Verification items for the finished model (mm, model axes). Coordinates: 2 decimals unless noted, no trailing zeros. Order: outer loops, then holes, each group sorted by start corner. A loop starts at its lowest first (then second) coordinate and runs counter-clockwise, first axis right, second up. Notation, with made-up numbers: M 43,-31 L 73,-31 A32 cw 73,-1 Z; hole C 68,43.5 d10. An arc over 180 degrees is marked long. Return JSON: item names as keys, results as strings. Group by question number.
Q1. Go/stop test with flat-tipped pins: pin 1 Ø1.8 at (y, z) = (-17, 348) entering from +X; pin 2 Ø1.3 at (y, z) = (-17, 348) entering from -X; pin 3 Ø1.3 at (x, y) = (-2.5, -16.5) entering from -Z. Record where each tip stops, or that it passes through.
Q2. Thickness scan on probe 1 along X at (y, z) = (-6.5, 83); probe 2 along Y at (x, z) = (2, 334). Record the ranges inside material, lowest first.
Q3. Section check B-B, the plane y = 7. Enter the section's corners in (x, z), then the cut area to 3 significant figures.
Q4. Section check A-A, the plane x = -3. Enter the section's corners in (y, z).
Q5. Section check C-C, the plane z = 30. Enter the section's corners in (x, y), then the cut area to 3 significant figures.
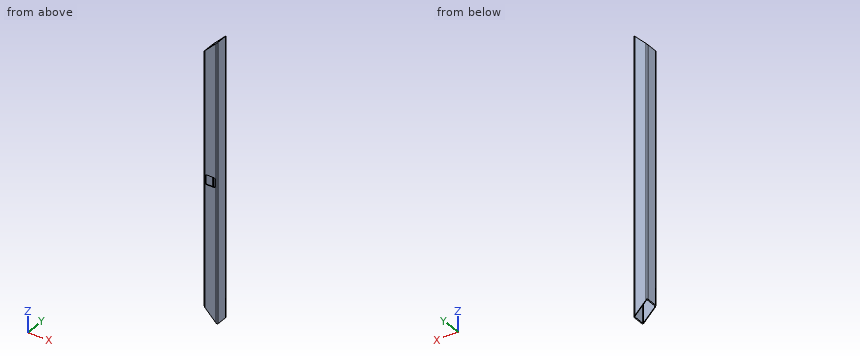
Autodesk Inventor part; units mm, degrees
ref_plane "Start plane" through (0, 0, -17.5) normal (0, 0, 1) x (1, 0, 0)
ref_plane "End plane" through (0, 0, 705.5) normal (0, 0, 1) x (1, 0, 0)
ref_plane "Work Plane4" through (0, 0, 344) normal (0, -1, 0) x (1, 0, 0)
ref_plane "Start plane" through (0, 0, -17.5) normal (0, 0, 1) x (1, 0, 0)
ref_plane "End plane" through (0, 0, 705.5) normal (0, 0, 1) x (1, 0, 0)
sketch "Sketch" plane through (0, 0, 0) normal (0, 0, 1) x (1, 0, 0)
  line L0 (-17.5, -14.3) -> (-17.5, 14.3)
  line L1 (-14.3, 17.5) -> (14.3, 17.5)
  line L2 (17.5, 14.3) -> (17.5, -14.3)
  line L3 (14.3, -17.5) -> (-14.3, -17.5)
  arc A0 (-17.5, -14.3) -> (-14.3, -17.5) centre (-14.3, -14.3) ccw
  arc A1 (-14.3, 17.5) -> (-17.5, 14.3) centre (-14.3, 14.3) ccw
  arc A2 (17.5, 14.3) -> (14.3, 17.5) centre (14.3, 14.3) ccw
  arc A3 (14.3, -17.5) -> (17.5, -14.3) centre (14.3, -14.3) ccw
  arc A4 (-14.3, 15.9) -> (-15.9, 14.3) centre (-14.3, 14.3) ccw
  line L4 (-14.3, 15.9) -> (14.3, 15.9)
  arc A5 (15.9, 14.3) -> (14.3, 15.9) centre (14.3, 14.3) ccw
  line L5 (15.9, 14.3) -> (15.9, -14.3)
  arc A6 (14.3, -15.9) -> (15.9, -14.3) centre (14.3, -14.3) ccw
  line L6 (14.3, -15.9) -> (-14.3, -15.9)
  arc A7 (-15.9, -14.3) -> (-14.3, -15.9) centre (-14.3, -14.3) ccw
  line L7 (-15.9, -14.3) -> (-15.9, 14.3)
  line L8 (0, 25.4278) -> (0, -25.4278) construction
  line L9 (-25.4278, 0) -> (25.4278, 0) construction
  dimension "d7" = 3.2
  dimension "d10" = 35
  dimension "d11" = 35
  dimension "d12" = 1.6
  dimension "d15" = 17.5
  dimension "d16" = 17.5
extrude "Body" add sketch "Sketch" along normal up to surface (723 mm away) from surface at -17.5
sketch "Sketch3" plane through (0, 0, 0) normal (0, 0, 1) x (1, 0, 0)
  line L0 (0, 0) -> (10, 0)
ref_plane "Work Plane3" through (0, 0, 0) normal (0, -1, 0) x (1, 0, 0)
sketch "Sketch4" plane through (0, 0, 0) normal (0, -1, 0) x (1, 0, 0)
  line L0 (-2, -17.5) -> (12, -17.5)
  line L1 (-2, 705.5) -> (12, 705.5)
  dimension "d18" = 723
ref_plane "Work Plane4" through (0, 0, 344) normal (0, -1, 0) x (1, 0, 0)
ref_plane "Work Plane5" through (0, -150, 344) normal (0, -1, 0) x (1, 0, 0)
ref_plane "Work Plane6" through (0, -75, 344) normal (0, -1, 0) x (1, 0, 0)
sketch "Sketch5" plane through (0, -75, 344) normal (0, -1, 0) x (1, 0, 0)
  arc A0 (-12.5, -9.3) -> (-9.3, -12.5) centre (-9.3, -9.3) ccw
  line L0 (-12.5, -9.3) -> (-12.5, 9.3)
  arc A1 (-9.3, 12.5) -> (-12.5, 9.3) centre (-9.3, 9.3) ccw
  line L1 (-9.3, 12.5) -> (9.3, 12.5)
  arc A2 (12.5, 9.3) -> (9.3, 12.5) centre (9.3, 9.3) ccw
  line L2 (12.5, 9.3) -> (12.5, -9.3)
  arc A3 (9.3, -12.5) -> (12.5, -9.3) centre (9.3, -9.3) ccw
  line L3 (9.3, -12.5) -> (-9.3, -12.5)
  arc A4 (-9.3, 10.9) -> (-10.9, 9.3) centre (-9.3, 9.3) ccw
  line L4 (-9.3, 10.9) -> (9.3, 10.9)
  arc A5 (10.9, 9.3) -> (9.3, 10.9) centre (9.3, 9.3) ccw
  line L5 (10.9, 9.3) -> (10.9, -9.3)
  arc A6 (9.3, -10.9) -> (10.9, -9.3) centre (9.3, -9.3) ccw
  line L6 (9.3, -10.9) -> (-9.3, -10.9)
  arc A7 (-10.9, -9.3) -> (-9.3, -10.9) centre (-9.3, -9.3) ccw
  line L7 (-10.9, -9.3) -> (-10.9, 9.3)
extrude "Extrusion2" cut sketch "Sketch5" along normal up to surface (150 mm away) from surface at -75 contours L0 A1 L1 A2 L2 A3 L3 A0 | L4 A5 L5 A6 L6 A7 L7 A4
ref_plane "Work Plane7" through (-17.5202, 0, 692.5586) normal (-0.871, 0, 0.4912) x (0.4912, 0, 0.871)
split "Split1" plane through (-17.5202, 0, 692.5586) removes the side toward (-0.871, 0, 0.4912)
ref_plane "Work Plane8" through (-17.5202, 0, -4.5586) normal (-0.871, 0, -0.4912) x (-0.4912, 0, 0.871)
split "Split2" plane through (-17.5202, 0, -4.5586) removes the side toward (-0.871, 0, -0.4912)
ref_plane "Work Plane9" through (17.5, 0, -17.5) normal (-0.7071, 0, -0.7071) x (-0.7071, 0, 0.7071)
split "Split3" plane through (17.5, 0, -17.5) removes the side toward (-0.7071, 0, -0.7071)
ref_plane "Work Plane10" through (17.5, 0, 705.5) normal (-0.7071, 0, 0.7071) x (0.7071, 0, 0.7071)
split "Split4" plane through (17.5, 0, 705.5) removes the side toward (-0.7071, 0, 0.7071)
equation "\"d7\" = G_IR"
equation "\"d10\" = G_H"
equation "\"d11\" = G_W"
equation "\"d12\" = G_T"
equation "\"d15\" = 0.5 * d10"
equation "\"d16\" = 0.5 * d11"
equation "\"d3\" = G_L"
equation "\"G_W\" = 35"
equation "\"G_H\" = 35"
equation "\"G_T\" = 1.6"
equation "\"G_IR\" = 3.2"
equation "\"G_L\" = d18"
equation "\"G_OFFSET_START\" = 17.5"
equation "\"G_OFFSET_END\" = 17.5"
equation "\"d13\" = -G_OFFSET_START"
equation "\"d14\" = G_OFFSET_END + B_L"
equation "\"B_L\" = 688"
properties part number "AS 1163 - C350L0 35x35x1.6 SHS - 723" material "Steel, Mild"
Numbers:
{
 "1": {"pin 1": "stops at x = 16.95", "pin 2": "stops at x = -16.76", "pin 3": "stops at z = 1.85"},
 "2": {"probe 1": "x = -17.5 to -15.9, 15.9 to 17.5", "probe 2": "y = 15.9 to 17.5"},
 "3": {"outline": "M -17.5,17.5 L -15.9,15.9 L -15.9,672.1 L -17.5,670.5 Z; M 15.9,-15.9 L 17.5,-17.5 L 17.5,705.5 L 15.9,703.9 Z", "area": "2,200 mm2"},
 "4": {"outline": "M -17.5,3 L -15.9,3 L -15.9,331.5 L -17.5,331.5 Z; M -17.5,356.5 L -15.9,356.5 L -15.9,685 L -17.5,685 Z; M 15.9,3 L 17.5,3 L 17.5,685 L 15.9,685 Z"},
 "5": {"outline": "M -17.5,-14.3 A3.2 ccw -14.3,-17.5 L 14.3,-17.5 A3.2 ccw 17.5,-14.3 L 17.5,14.3 A3.2 ccw 14.3,17.5 L -14.3,17.5 A3.2 ccw -17.5,14.3 Z; hole M -15.9,-14.3 A1.6 ccw -14.3,-15.9 L 14.3,-15.9 A1.6 ccw 15.9,-14.3 L 15.9,14.3 A1.6 ccw 14.3,15.9 L -14.3,15.9 A1.6 ccw -15.9,14.3 Z", "area": "207 mm2"}
}
